Source: CAD feature listing. Evaluate the final solid. Frame: model axes, mm. Face numbers are marked on the shaded views. A direction names the side the tool comes from. Give positions to 0.01 mm unless a question says otherwise; leave off trailing zeros. Order: outer loops, then holes, each group sorted by start corner. A loop starts at its lowest first (then second) coordinate and runs counter-clockwise, first axis right, second up.
Autodesk Inventor part; units mm, degrees
ref_plane "YZ Plane" through (0, 0, 0) normal (1, 0, 0) x (0, 1, 0)
ref_plane "XZ Plane" through (0, 0, 0) normal (0, 1, 0) x (-1, 0, 0)
ref_plane "XY Plane" through (0, 0, 0) normal (0, 0, 1) x (1, 0, 0)
sketch "Boceto1" plane through (0, 0, 0) normal (0, 1, 0) x (-1, 0, 0)
  line L0 (0, 0) -> (30, 0)
  line L1 (30, 0) -> (30, -30)
  line L2 (30, -30) -> (0, -30)
  line L3 (0, -30) -> (0, 0)
  circle A0 centre (15, -15) radius 4
  dimension "d0" = 30
  dimension "d1" = 30
  dimension "d2" = 8
extrude "Extrusión1" add sketch "Boceto1" along normal blind 50
sketch "Boceto2" plane through (0, 50, 0) normal (0, 1, 0) x (1, 0, 0)
  circle A0 centre (-15, 15) radius 4
  circle A1 centre (-15, 15) radius 15
  point P0 (0, 0)
  dimension "d5" = 30
extrude "Extrusión2" add sketch "Boceto2" along normal blind 5
sketch "Boceto3" plane through (0, 0, 0) normal (0, -1, 0) x (1, 0, 0)
  circle A0 centre (-15, -15) radius 4
  circle A1 centre (-15, -15) radius 5.5
  line L0 (-2, -28) -> (-28, -28)
  line L1 (-28, -28) -> (-28, -2)
  line L2 (-28, -2) -> (-2, -2)
  line L3 (-2, -2) -> (-2, -28)
  line L4 (-2, -28) -> (-28, -2) construction
  line L5 (-28, -28) -> (-2, -2) construction
  point P0 (0, 0)
  dimension "d8" = 11
  dimension "d9" = 26
  dimension "d10" = 26
extrude "Extrusión3" cut sketch "Boceto3" against normal blind 46 contours L0 L1 L2 L3
properties part number "Troncox1"
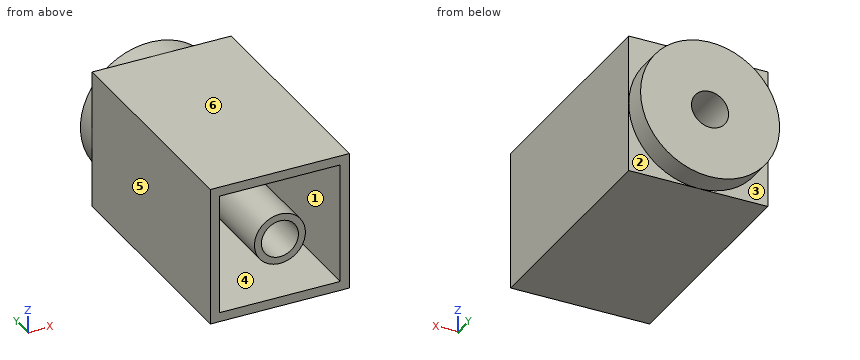
1) Section query C-C on z = -23. Output: boundary loops of the cut face in (x, y).
Checks:
outline: (-30, 0) - (-28, 0) - (-28, 46) - (-2, 46) - (-2, 0) - (0, 0) - (0, 50) - (-2.31, 50) - (-2.31, 55) - (-27.69, 55) - (-27.69, 50) - (-30, 50) - close
2) Ray query, L1, parallel to Z at x = -15, y = 36; L2, parallel to X at y = 40, z = -8. Return the intervals inside material, ascending.
Checks:
L1: z = -30 to -28, -20.5 to -19, -11 to -9.5, -2 to 0
L2: x = -30 to -28, -2 to 0
3) Section query A-A on y = 7.5. Output: boundary loops of the cut face in (x, z), and give its area (3 significant figures).
Checks:
outline: (-30, -30) - (0, -30) - (0, 0) - (-30, 0) - close; circle Ø11 at (-15, -15); hole (-28, -28) - (-2, -28) - (-2, -2) - (-28, -2) - close; hole circle Ø8 at (-15, -15)
area: 269 mm2
4) Pull-direction query (Z, two-part tool) for the marked faces 4, 5 and 6; classes: +Z half, -Z half, draft (parallel to the pull), parting line (faces both ways), or undercut.
Checks:
face 4: undercut
face 5: draft
face 6: +Z half
5) Reachability of the marked faces 1, 2 and 3 from +Z, -Z, +X, -X, +Y, -Y: full face, straight path, thin tool, end or side. Return the list, or none.
Checks:
face 1: -Y
face 2: -Z, +X, +Y
face 3: -Z, -X, +Y
6) First-contact query: pin 1 Ø3 at (x, y) = (-24, 37) entering from +Z; pin 2 Ø3 at (x, z) = (-11.5, -24.5) entering from -Y. Flat tips, straight axial feed; report the tip coordinate or a pass-through.
Checks:
pin 1: stops at z = 0
pin 2: stops at y = 46
7) Section query B-B on x = -3. Output: boundary loops of the cut face in (y, z), and give its area (3 significant figures).
Checks:
outline: (0, -30) - (50, -30) - (50, -24) - (55, -24) - (55, -6) - (50, -6) - (50, 0) - (0, 0) - (0, -2) - (46, -2) - (46, -28) - (0, -28) - close
area: 394 mm2
